Geometry: final body of the model. Coordinates: model frame, mm. Coordinates: 2 decimals unless noted, no trailing zeros. Order: outer loops, then holes, each group sorted by start corner. A loop starts at its lowest first (then second) coordinate and runs counter-clockwise, first axis right, second up. Notation, with made-up numbers: (86.5, 71) -> (123.5, 71) arc R26 cw to (123.5, 97) -> close; hole circle Ø11 at (83, -21.5). An arc over 180 degrees is marked (long way). Answer in a Markdown table with one row per item. Add a question column.
1) Section query A-A on z = 25. Return the cut outline in (x, y).
2) Section query B-B on y = 38.5. Return the cut outline in (x, z), then the cut area to 3 significant figures.
3) Pull-direction query (Z, two-part tool) for faces 1 (the face through (0.07, 37.198, 34.915)), 2 (the face through (0, 123, 40)), 3 (the face through (5, 123, -1)); classes: +Z half, -Z half, draft (parallel to the pull), parting line (faces both ways), or undercut.
4) Section query C-C on x = 2. Return the cut outline in (y, z), then the cut area to 3 significant figures.
5) Ray query, line 1 (Z direction, x = -1.75, y = 38.5); line 2 (Y direction, x = -4, z = 26); line 3 (Z direction, x = -1.5, y = 30.5). Return the intervals inside material, ascending. Write a range as from..to.
```python
from build123d import *

# Parameters (mm, degrees)
F0_W     = 10
F0_H     = 80
F1_DEPTH = 250
F2_R     = 10
F3_DEPTH = 10.001


with BuildPart() as f1:
    # F0 (on Front) → F1 (new body)
    with BuildSketch(Plane.XZ):
        Rectangle(F0_W, F0_H)
    extrude(amount=-F1_DEPTH)

    # F2 (on face) → F3 (cut, through all)
    with BuildSketch(Plane.YZ.offset(5)):
        with Locations((38.5, 25)):
            Circle(F2_R)
    extrude(amount=-F3_DEPTH, mode=Mode.SUBTRACT)


solid = f1.part
```
Result:
| question | item | result |
|---|---|---|
| 1 | outline | (-5, 0) -> (5, 0) -> (5, 28.5) -> (-5, 28.5) -> close; (-5, 48.5) -> (5, 48.5) -> (5, 250) -> (-5, 250) -> close |
| 2 | outline | (-5, -40) -> (5, -40) -> (5, 15) -> (-5, 15) -> close; (-5, 35) -> (5, 35) -> (5, 40) -> (-5, 40) -> close |
| 2 | area | 600 mm2 |
| 3 | face 1 | undercut |
| 3 | face 2 | +Z half |
| 3 | face 3 | draft |
| 4 | outline | (0, -40) -> (250, -40) -> (250, 40) -> (0, 40) -> close; hole circle Ø20 at (38.5, 25) |
| 4 | area | 19,700 mm2 |
| 5 | line 1 | -40..15, 35..40 |
| 5 | line 2 | 0..28.55, 48.45..250 |
| 5 | line 3 | -40..19, 31..40 |
